Autodesk Inventor part; units mm, degrees
ref_plane "YZ Plane" through (0, 0, 0) normal (1, 0, 0) x (0, 1, 0)
ref_plane "XZ Plane" through (0, 0, 0) normal (0, 1, 0) x (-1, 0, 0)
ref_plane "XY Plane" through (0, 0, 0) normal (0, 0, 1) x (1, 0, 0)
ref_plane "Work Plane1" through (0, 0, 0) normal (0, 0, -1) x (-1, 0, 0)
sketch "Sketch20" plane through (0, 0, 0) normal (0, 0, -1) x (-1, 0, 0)
  line L0 (0, 0) -> (25.4, 0)
  line L1 (25.4, 0) -> (0, 0)
  line L2 (0, 0) -> (0, 50.8)
  line L3 (0, 50.8) -> (25.4, 50.8)
  line L4 (25.4, 50.8) -> (25.4, 0)
  line L5 (23.749, 49.149) -> (1.651, 49.149)
  line L6 (1.651, 49.149) -> (1.651, 1.651)
  line L7 (1.651, 1.651) -> (23.749, 1.651)
  line L8 (23.749, 1.651) -> (23.749, 49.149)
  line L9 (0, 0) -> (0, 50.8)
  dimension "d71" = 25.4
  dimension "d72" = 50.8
  dimension "d73" = 1.651
  dimension "d74" = 1.651
  dimension "d75" = 1.651
  dimension "d76" = 1.651
  dimension "d78" = 0
extrude "Extrusion16" add sketch "Sketch20" against normal blind 152.4
ref_plane "Work Plane4" through (76.2, 0, 0) normal (0, -1, 0) x (1, 0, 0)
sketch "Sketch21" plane through (76.2, 0, 0) normal (0, -1, 0) x (1, 0, 0)
  circle A0 centre (-38.1, 12.7) radius 2.5797
  circle A1 centre (-63.5, 12.7) radius 2.5797
  circle A2 centre (-88.9, 12.7) radius 2.5797
  circle A3 centre (-88.9, 38.1) radius 2.5797
  circle A4 centre (-88.9, 63.5) radius 2.5797
  line L0 (-76.2, 25.4) -> (0, 25.4)
  line L1 (-101.6, 0) -> (-101.6, 152.4)
  line L2 (-76.2, 25.4) -> (-76.2, 152.4)
  point P0 (-76.2, 0)
  dimension "d81" = 12.7
  dimension "d82" = 12.7
  dimension "d83" = 12.7
  dimension "d84" = 25.4
  dimension "d85" = 12.7
  dimension "d86" = 5.1594
  dimension "d87" = 5.1594
  dimension "d88" = 5.1594
  dimension "d89" = 25.4
  dimension "d90" = 25.4
  dimension "d91" = 25.4
  dimension "d92" = 5.1594
  dimension "d93" = 5.1594
  dimension "d94" = 12.7
  dimension "d95" = 12.7
extrude "Extrusion17" cut sketch "Sketch21" against normal blind 76.2
ref_plane "Work Plane3" through (-25.4, 0, 0) normal (-1, 0, 0) x (0, 0, 1)
sketch "Sketch26" plane through (-25.4, 0, 0) normal (-1, 0, 0) x (0, 0, 1)
  circle A0 centre (107.569, 38.1) radius 2.5797
  line L0 (152.4, 50.8) -> (152.4, 0)
  line L1 (0, 50.8) -> (152.4, 50.8)
  circle A1 centre (47.752, 38.1) radius 2.5797
  circle A2 centre (107.569, 12.7) radius 2.5797
  circle A3 centre (47.752, 12.7) radius 2.5797
  point P0 (0, 0)
  dimension "d122" = 5.1594
  dimension "d123" = 44.831
  dimension "d124" = 12.7
  dimension "d125" = 5.1594
  dimension "d126" = 59.817
  dimension "d129" = 25.4
  dimension "d130" = 5.1594
  dimension "d131" = 25.4
  dimension "d132" = 5.1594
  dimension "d143" = 12.7
extrude "Extrusion22" cut sketch "Sketch26" against normal blind 25.4
ref_plane "Work Plane2" through (76.2, 50.8, 25.4) normal (0, 1, 0) x (1, 0, 0)
sketch "Sketch27" plane through (76.2, 50.8, 25.4) normal (0, 1, 0) x (1, 0, 0)
  circle A0 centre (-88.9, -114.3) radius 2.5797
  circle A1 centre (-88.9, -88.9) radius 2.5797
  line L0 (-76.2, -127) -> (-101.6, -127)
  line L1 (-76.2, 0) -> (-76.2, -127)
  point P0 (-76.2, 25.4)
  dimension "d135" = 12.7
  dimension "d136" = 12.7
  dimension "d137" = 38.1
  dimension "d138" = 12.7
  dimension "d139" = 5.1594
  dimension "d140" = 5.1594
extrude "Extrusion23" cut sketch "Sketch27" against normal blind 50.8
equation "\"d74\" = d73"
equation "\"d75\" = d73"
equation "\"d76\" = d73"
equation "\"d87\" = d86"
equation "\"d88\" = d86"
equation "\"d92\" = d86"
equation "\"d93\" = d86"
equation "\"d125\" = d122"
equation "\"d130\" = d122"
equation "\"d132\" = d122"
equation "\"d140\" = d139"
properties part number "left arm"
The listing builds one solid part. Answer for the finished solid, in the listing's coordinates (mm). A direction names the side the tool comes from. Coordinates: 2 decimals unless noted, no trailing zeros. Order: outer loops, then holes, each group sorted by start corner. A loop starts at its lowest first (then second) coordinate and runs counter-clockwise, first axis right, second up. Notation, with made-up numbers: (73, 68) -> (79, 68) arc R11 cw to (79, 87) -> close; hole circle Ø4 at (-39.75, 53). An arc over 180 degrees is marked (long way). Answer in a Markdown table with one row per item. Add a question column.
Item 1: Find the intervals of material crossed by L1, parallel to Z at x = -12.7, y = 1.15; L2, parallel to Y at x = -5, z = 89.5; L3, parallel to X at y = 36.5, z = 54, in increasing order. Write a range as from..to.
Item 2: Find section B-B (y = 38.1). Write down the section's boundary in (x, z), then the cut area to 3 significant figures.
Item 3: Find section C-C (z = 24). Write down the section's boundary in (x, y).
Item 4: Find section A-A (x = -18). Write down the section's boundary in (y, z), then the cut area to 3 significant figures.
Item 5: Determine the mould class of faces 3 (the face through (-13, 49.149, 75)), 4 (the face through (-13, 50.8, 75)), 5 (the face through (-10.317, 49.963, 11.712)), 6 (the face through (0, 25, 75)) for opening direction X: +X half, -X half, draft (parallel to the pull), parting line (faces both ways), or undercut.
Item 6: Find section D-D (y = 27.5). Write down the section's boundary in (x, z).
Item 7: This flat-tipped pin is pushed along its axis until it touches: P1, Ø4, axis at y = 38.1, z = 47.752, coming from the -X side. Where does it stop, or does it pass through?
Item 8: Which of the six approach directions +Z, -Z, +X, -X, +Y, -Y give full straight-line access (tool end or side, diameter ignored) to faces 1 (the face through (-11.313, 0.814, 65.675)), 2 (the face through (-13, 1.651, 75))?
Result set:
| question | item | result |
|---|---|---|
| 1 | L1 | z = 0..10.12, 15.28..35.52, 40.68..60.92, 66.08..111.72, 116.88..137.12, 142.28..152.4 |
| 1 | L2 | y = 0..1.65, 49.15..50.8 |
| 1 | L3 | x = -25.4..-23.75, -1.65..0 |
| 2 | outline | (-25.4, 0) -> (-23.75, 0) -> (-23.75, 45.17) -> (-25.4, 45.17) -> close; (-25.4, 50.33) -> (-23.75, 50.33) -> (-23.75, 104.99) -> (-25.4, 104.99) -> close; (-25.4, 110.15) -> (-23.75, 110.15) -> (-23.75, 152.4) -> (-25.4, 152.4) -> close; (-1.65, 0) -> (0, 0) -> (0, 45.17) -> (-1.65, 45.17) -> close; (-1.65, 50.33) -> (0, 50.33) -> (0, 104.99) -> (-1.65, 104.99) -> close; (-1.65, 110.15) -> (0, 110.15) -> (0, 152.4) -> (-1.65, 152.4) -> close |
| 2 | area | 469 mm² |
| 3 | outline | (-25.4, 0) -> (0, 0) -> (0, 50.8) -> (-25.4, 50.8) -> close; hole (-23.75, 1.65) -> (-1.65, 1.65) -> (-1.65, 49.15) -> (-23.75, 49.15) -> close |
| 4 | outline | (0, 0) -> (1.65, 0) -> (1.65, 152.4) -> (0, 152.4) -> close; (49.15, 0) -> (50.8, 0) -> (50.8, 152.4) -> (49.15, 152.4) -> close |
| 4 | area | 503 mm² |
| 5 | face 3 | undercut |
| 5 | face 4 | draft |
| 5 | face 5 | undercut |
| 5 | face 6 | +X half |
| 6 | outline | (-25.4, 0) -> (-23.75, 0) -> (-23.75, 152.4) -> (-25.4, 152.4) -> close; (-1.65, 0) -> (0, 0) -> (0, 152.4) -> (-1.65, 152.4) -> close |
| 7 | P1 | passes through |
| 8 | face 1 | +Y, -Y |
| 8 | face 2 | +Z, -Z |
